Can you work these out from the model? Positions are in its coordinate system, mm. Face numbers are marked on the shaded views. A direction names the side the tool comes from. Give positions to 0.01 mm unless a question says otherwise; leave off trailing zeros. Loops run counter-clockwise (first coordinate to the right, second up) from the corner with the lowest first, then second, coordinate; pieces in that order, holes last. Notation, with made-up numbers: M -2.5,74.5 L 30.5,74.5 A16 cw 30.5,89.5 Z; hole C -11,-24.5 d7. An arc over 180 degrees is marked long. Answer as a JSON object with one key per item and string values.
Autodesk Inventor part; units mm, degrees
ref_plane "YZ Plane" through (0, 0, 0) normal (1, 0, 0) x (0, 1, 0)
ref_plane "XZ Plane" through (0, 0, 0) normal (0, 1, 0) x (-1, 0, 0)
ref_plane "XY Plane" through (0, 0, 0) normal (0, 0, 1) x (1, 0, 0)
sketch "Esboço1" plane through (0, 0, 0) normal (0, 1, 0) x (-1, 0, 0)
  line L0 (0, 0) -> (25, 0)
  line L1 (25, 0) -> (25, -30)
  line L2 (25, -30) -> (0, -30)
  line L3 (0, -30) -> (0, 0)
  dimension "d0" = 25
  dimension "d1" = 30
extrude "Extrusão1" add sketch "Esboço1" along normal blind 20
sketch "Esboço2" plane through (0, 20, 0) normal (0, 1, 0) x (1, 0, 0)
  line L0 (0, 30) -> (-25, 30)
  line L1 (-25, 30) -> (-25, 0)
  line L2 (-25, 0) -> (0, 0)
  point P0 (-12.5, 7.5)
  point P1 (-12.5, 22.5)
  point P2 (-12.5, 30)
  point P3 (-12.5, 0)
  dimension "d4" = 25
  dimension "d5" = 12.5
  dimension "d6" = 12.5
  dimension "d31" = 7.5
  dimension "d32" = 7.5
hole "Furo1" at (-12.5, 20, -7.5) at (-12.5, 20, -22.5) direction (0, -1, 0) diameter 4.134 depth 14.2 tip angle 118
sketch "Esboço3" plane through (0, 0, 0) normal (0, -1, 0) x (1, 0, 0)
  circle A0 centre (-12.5, -15) radius 7.5 construction
  line L0 (0, 0) -> (0, -30)
  line L1 (0, -30) -> (-25, -30)
  line L2 (-25, -30) -> (-25, 0)
  line L3 (0, -30) -> (-25, -30)
  line L4 (0, 0) -> (0, -30)
  line L5 (-25, 0) -> (0, 0)
  dimension "d16" = 25
  dimension "d17" = 30
  dimension "d18" = 12.5
  dimension "d19" = 15
  dimension "d21" = 15
extrude "Extrusão2" add sketch "Esboço3" along normal blind 20
sketch "Esboço5" plane through (-12.5, -20, -15) normal (0, -1, 0) x (1, 0, 0)
  circle A0 centre (0, 0) radius 7.5
  point P0 (12.5, 15)
hole "Furo3" at (-12.5, -20, -15) direction (0, 1, 0) diameter 8.376 depth 20 tip angle 118
equation "\"d18\" = 0.5 * d16"
equation "\"d19\" = 0.5 * d17"
equation "\"Raio_vergadura\" = Espessura"
equation "\"Largura_alívio_de_vergadura\" = Espessura"
equation "\"Profundidade_alívio_de_vergadura\" = 0.5 * Espessura"
equation "\"Tamanho_alívio_de_dobra\" = 4 * Espessura"
equation "\"Remanescente_mínimo\" = 2 * Espessura"
equation "\"Raiodetransição\" = Raio_vergadura"
equation "\"Tamanho_de_raio_de_Jacobi\" = Raio_vergadura"
equation "\"TamanhoFolga\" = Espessura"
properties part number "Suporte da probe" material "Alumínio 6061"
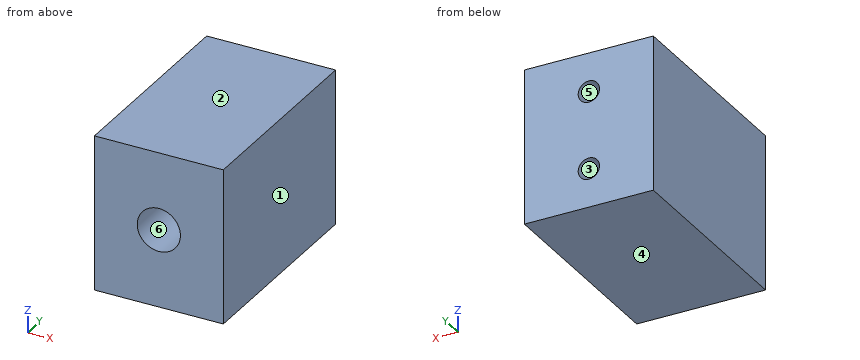
1) Suppose I cut it at A-A, the plane y = -4. Write out the boundary of the cut face in (x, z).
Answer list:
{"outline": "M -25,-30 L 0,-30 L 0,0 L -25,0 Z; hole C -12.5,-15 d8.38"}
2) For the marked faces 4, 5 and 6, which set-ups out of +Z, -Z, +X, -X, +Y, -Y let a thin tool reach every point of the face, with its end or its side?
Answer list:
{"face 4": "-Z, +X, -X, +Y, -Y", "face 5": "+Y", "face 6": "-Y"}
3) Please list where these lines run through material, in increasing order: line 1 along Z through (x, y) = (-12.5, 14.5); line 2 along X through (y, z) = (10, -22.5); line 3 along X through (y, z) = (-14.75, -15). Write a range as from..to.
Answer list:
{"line 1": "-30..-24.57, -20.43..-9.57, -5.43..0", "line 2": "-25..-14.57, -10.43..0", "line 3": "-25..-16.69, -8.31..0"}
4) If we mould it in two halves opening along X, with no side actions, what happens to the marked faces 1, 2 and 3? For each: +X half, -X half, draft (parallel to the pull), parting line (faces both ways), or undercut.
Answer list:
{"face 1": "+X half", "face 2": "draft", "face 3": "undercut"}
5) Will these pins go through, and if not, where does the flat tip stop? pin 1 Ø1 at (y, z) = (-4, -8.5) entering from +X; pin 2 Ø3.5 at (x, z) = (-12.5, -22.5) entering from +Y.
Answer list:
{"pin 1": "x = 0", "pin 2": "y = 5.61"}
